from build123d import *

# Parameters (mm, degrees)
F1_DEPTH = 63.5
F2_DEPTH = 38.1
F3_DEPTH = 31.75


with BuildPart() as f1:
    # F0 (on Front) → F1 (new body, symmetric)
    with BuildSketch(Plane.XZ):
        Polygon((22.225, 9.525), (-41.275, 9.525), (-41.275, -9.525), (41.275, -9.525), (41.275, 9.525), align=None)
    extrude(amount=F1_DEPTH, both=True)

    # F0 (on Front) → F2 (join, symmetric)
    with BuildSketch(Plane.XZ):
        with BuildLine():
            Line((22.225, 47.863565), (22.225, 9.525))
            Line((22.225, 9.525), (41.275, 9.525))
            Line((41.275, 9.525), (41.275, 47.863565))
            ThreePointArc((41.275, 47.863565), (43.886262, 58.190434), (51.092341, 66.034881))
            Line((51.092341, 66.034881), (95.982485, 66.034881))
            Line((95.982485, 66.034881), (95.982485, 85.084881))
            Line((95.982485, 85.084881), (46.350457, 85.084881))
            ThreePointArc((46.350457, 85.084881), (28.783869, 70.041618), (22.225, 47.863565))
        make_face()
    extrude(amount=F2_DEPTH, both=True)

    # F0 (on Front) → F3 (join, symmetric)
    with BuildSketch(Plane.XZ):
        with BuildLine():
            add(Edge.make_bspline(
                [(-41.275, 9.525), (-6.610331, 19.785214), (0, 84.11859), (46.350457, 85.084881)],
                knots=[0, 0, 0, 0, 115.704435, 115.704435, 115.704435, 115.704435], degree=3))
            Line((-41.275, 9.525), (22.225, 9.525))
            Line((22.225, 9.525), (22.225, 47.863565))
            ThreePointArc((22.225, 47.863565), (28.783869, 70.041618), (46.350457, 85.084881))
        make_face()
    extrude(amount=F3_DEPTH, both=True)

    # F0 (on Front) → F4 (revolve)
    with BuildSketch(Plane.XZ):
        Polygon((95.982485, 88.993471), (95.982485, 85.084881), (95.982485, 66.034881), (95.982485, 54.514322), (140.712164, 54.514322), (140.712164, 88.993471), align=None)
    revolve(axis=Axis((95.982485, 0, 71.753897), (0, 0, 1)))


solid = f1.part
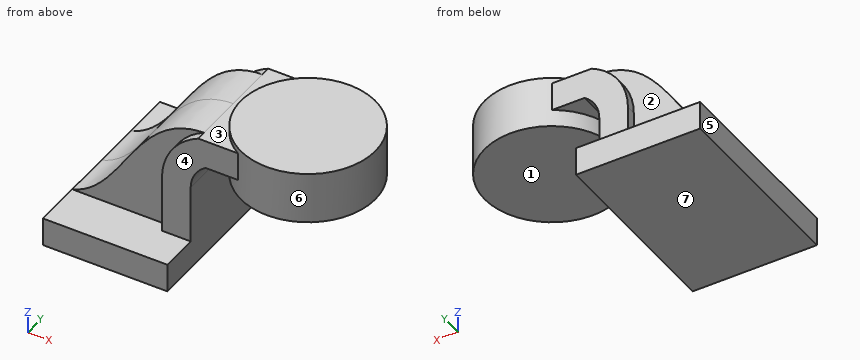
Design review of the part built by this model. Coordinates are the model's own, in mm. Face numbers are marked on the shaded views. A direction names the side the tool comes from. Give positions to 0.01 mm unless a question says otherwise; leave off trailing zeros. Loops run counter-clockwise (first coordinate to the right, second up) from the corner with the lowest first, then second, coordinate; pieces in that order, holes last. Notation, with made-up numbers: (32.25, -4) - (90.25, -4) arc R11 ccw to (90.25, 0) - close; hole circle Ø10 at (77, 24). An arc over 180 degrees is marked (long way). Use CSV: the item, a comma, the result in double quotes. Start each with the question number.
1. Machinability: for the marked faces 1, 2, 3 and 4, which of the approach directions +Z, -Z, +X, -X, +Y, -Y give a long, thin tool a straight path to every point of the face, cutting with its end or side? Answer none if there is none.
2. Add section B-B (x = 99). State the section outline as (y, z) points, plus the area to 3 significant figures.
3. Wall thickness on L1, parallel to X at y = -25.5, z = 4 (3 decimals); L2, parallel to Z at x = 60, y = 13.5; L3, parallel to Y at x = 16, z = 21.5: over which ranges is each line inside the solid? List them lowest first.
4. Add section C-C (x = 78). State the section outline as (y, z) points, plus the area to 3 significant figures.
5. Add section A-A (y = 41). State the section outline as (x, z) points (3 decimals).
6. Insertion check: P1, Ø10, axis at x = 103, z = 71, coming from the +Y side; P2, Ø4, axis at x = 78, z = 67.5, coming from the -Y side; P3, Ø16, axis at x = -19.5, y = -40, coming from the +Z side (3 decimals). Each pin has a flat end and moves straight along its axis. Give the tip position at first contact, or say it passes through.
7. Draft analysis for pull direction X (two halves, no side actions). For the marked faces 5, 6 and 7, state which applies: released by +X, released by -X, zero draft, split by the parting line, or undercut.
Results found:
1,face 1,"-Z, +X, +Y, -Y"
1,face 2,"+Z, -X, +Y"
1,face 3,"+Z, -X"
1,face 4,"+Z, -X, -Y"
2,outline,"(-44.63, 54.51) - (44.63, 54.51) - (44.63, 88.99) - (-44.63, 88.99) - close"
2,area,"3,080 mm²"
3,L1,"x = -41.275 to 41.275"
3,L2,"z = 54.51 to 88.99"
3,L3,"y = -31.75 to 31.75"
4,outline,"(-40.96, 54.51) - (40.96, 54.51) - (40.96, 88.99) - (-40.96, 88.99) - close"
4,area,"2,820 mm²"
5,outline,"(-41.275, -9.525) - (41.275, -9.525) - (41.275, 9.525) - (-41.275, 9.525) - close; (78.101, 54.514) - (113.864, 54.514) - (113.864, 88.993) - (78.101, 88.993) - close"
6,P1,"stops at y = 44.68"
6,P2,"stops at y = -41.78"
6,P3,"stops at z = 9.525"
7,face 5,"released by -X"
7,face 6,"undercut"
7,face 7,"zero draft"
